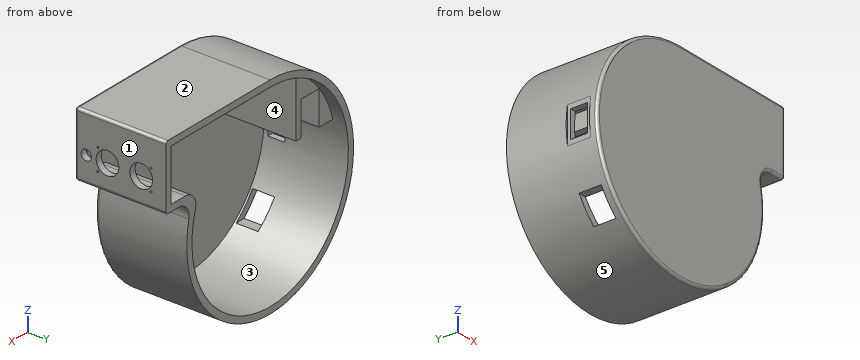
```python
from build123d import *

# Parameters (mm, degrees)
BOSS_EXTRUDE1_DEPTH     = 70
SHELL1_T                = -5
SKETCH3_R               = 8.75
SKETCH3_R_2             = 0.75
SKETCH3_R_3             = 4
CUT_EXTRUDE1_DEPTH      = 5
CUT_EXTRUDE2_REACH      = 147.945
CUT_EXTRUDE2_END_RADIUS = 80
SKETCH4_W               = 17
SKETCH4_H               = 17
SKETCH4_W_2             = 21
SKETCH4_H_2             = 13
CUT_EXTRUDE3_DEPTH      = 146.945195193
CUT_EXTRUDE3_DEPTH_BACK = 146.945195193
SKETCH5_W               = 2.5
SKETCH5_H               = 18
BOSS_EXTRUDE3_DEPTH     = 55
FILLET1_R               = 10
FILLET2_R               = 2


with BuildPart() as part:
    # Sketch1 → Boss-Extrude1 (new body)
    with BuildSketch(Plane(origin=(0, 0, 0), x_dir=(1, 0, 0), z_dir=(0, 1, 0))):
        with BuildLine():
            Line((0, -80), (100, -80))
            Line((100, -80), (100, -30))
            Line((100, -30), (74.161984871, -30))
            ThreePointArc((74.161984871, -30), (-44.72135955, 66.332495807), (0, -80))
        make_face()
    extrude(amount=BOSS_EXTRUDE1_DEPTH)

    # Shell1
    shell1_openings = [part.faces().sort_by_distance(p)[0] for p in [
        (7.618956149, 70, 6.200850369),
    ]]
    offset(amount=SHELL1_T, openings=shell1_openings, kind=Kind.INTERSECTION)

    # Sketch3 → Cut-Extrude1 (cut)
    with BuildSketch(Plane(origin=(100, 0, 0), x_dir=(0, 0, -1), z_dir=(1, 0, 0))):
        with Locations((-50, 25)):
            Circle(SKETCH3_R)
        with Locations((-50, 51)):
            Circle(SKETCH3_R)
        with Locations((-41.75, 58.5)):
            Circle(SKETCH3_R_2)
        with Locations((-41.75, 17.5)):
            Circle(SKETCH3_R_2)
        with Locations((-58.25, 17.5)):
            Circle(SKETCH3_R_2)
        with Locations((-58.25, 58.5)):
            Circle(SKETCH3_R_2)
        with Locations((-50, 8.65)):
            Circle(SKETCH3_R_3)
    extrude(amount=-CUT_EXTRUDE1_DEPTH, mode=Mode.SUBTRACT)

    # Cut-Extrude2: up to this cylinder (the profile starts inside it)
    cut_extrude2_end = Plane(origin=(0, 15, 0), z_dir=(0, -1, 0)) * Cylinder(CUT_EXTRUDE2_END_RADIUS, 456.89, mode=Mode.PRIVATE)
    # Sketch4 → Cut-Extrude2 (cut, up to the surface)
    with BuildSketch(Plane(origin=(0, 0, 0), x_dir=(0, 0, -1), z_dir=(1, 0, 0)), mode=Mode.PRIVATE) as cut_extrude2_sk1:
        with Locations((50.5, 15)):
            Rectangle(SKETCH4_W, SKETCH4_H)
    cut_extrude2_tool1 = extrude(cut_extrude2_sk1.sketch, amount=-CUT_EXTRUDE2_REACH, mode=Mode.PRIVATE) & cut_extrude2_end
    add(cut_extrude2_tool1.solids().sort_by_distance((0, 15, -50.5))[0], mode=Mode.SUBTRACT)
    # Sketch4 → Cut-Extrude2 (cut, up to the surface)
    with BuildSketch(Plane(origin=(0, 0, 0), x_dir=(0, 0, -1), z_dir=(1, 0, 0)), mode=Mode.PRIVATE) as cut_extrude2_sk2:
        with Locations((0, 15)):
            Rectangle(SKETCH4_W_2, SKETCH4_H_2)
    cut_extrude2_tool2 = extrude(cut_extrude2_sk2.sketch, amount=-CUT_EXTRUDE2_REACH, mode=Mode.PRIVATE) & cut_extrude2_end
    add(cut_extrude2_tool2.solids().sort_by_distance((0, 15, 0))[0], mode=Mode.SUBTRACT)

    # Sketch5 → Cut-Extrude3 (cut, two sides: drawn at the far end of the back side and taken through both)
    with BuildSketch(Plane.XY.offset(-CUT_EXTRUDE3_DEPTH_BACK)):
        with Locations((-79.998342826, 15)):
            Rectangle(SKETCH5_W, SKETCH5_H)
    extrude(amount=CUT_EXTRUDE3_DEPTH + CUT_EXTRUDE3_DEPTH_BACK, mode=Mode.SUBTRACT)

    # Sketch6 → Boss-Extrude3 (add)
    with BuildSketch(Plane(origin=(0, 5, 0), x_dir=(1, 0, 0), z_dir=(0, 1, 0))):
        with BuildLine():
            Line((-72.5176701, -19.136026841), (-59.5176701, -19.136026841))
            Line((-59.5176701, -19.136026841), (-59.5176701, -45.636026841))
            Line((-59.5176701, -45.636026841), (-42.0176701, -45.636026841))
            Line((-42.0176701, -45.636026841), (-42.0176701, -19.136026841))
            Line((-42.0176701, -19.136026841), (-37.0176701, -19.136026841))
            Line((-37.0176701, -19.136026841), (-37.0176701, -65.228000892))
            Line((-37.0176701, -65.228000892), (-37.0176701, -67.228000892))
            ThreePointArc((-37.0176701, -67.228000892), (-61.280154536, -47.480406071), (-74.5176701, -19.136026841))
            Line((-74.5176701, -19.136026841), (-72.5176701, -19.136026841))
        make_face()
    extrude(amount=BOSS_EXTRUDE3_DEPTH)

    # Fillet1
    fillet1_edges = [part.edges().sort_by_distance(p)[0] for p in [
        (66.332495807, 37.5, 35),
        (74.161984871, 35, 30),
    ]]
    fillet(fillet1_edges, radius=FILLET1_R)

    # Fillet2
    fillet2_edges = [part.edges().sort_by_distance(p)[0] for p in [
        (-49.888765157, 0, -62.538876798),
        (79.932284274, 0, 26.236095645),
        (93.874821937, 0, 30),
        (100, 0, 55),
        (50, 0, 80),
        (100, 35, 30),
        (100, 35, 80),
    ]]
    fillet(fillet2_edges, radius=FILLET2_R)


solid = part.part
```
Part model, mm, in its own coordinate system. Face numbers are marked on the shaded views. A direction names the side the tool comes from. Round coordinates to 2 decimals unless told otherwise and drop trailing zeros. Loops run counter-clockwise (first coordinate to the right, second up) from the corner with the lowest first, then second, coordinate; pieces in that order, holes last.
Item 1: 3-axis set-ups, long thin cutter, end or side, ignore diameter. For the marked faces 4 and 5: which of +Z, -Z, +X, -X, +Y, -Y reach the whole face in a straight line?
Item 2: Cut at B-B, the plane y = 48.5. Give the cut face in (x, z).
Item 3: Drop flat-ended pins along their axis: P1, Ø9, axis at x = -50, y = 26.5, coming from the -Z side; P2, Ø5, axis at x = 32.5, z = 1, coming from the +Y side; P3, Ø7, axis at y = 8.65, z = 50, coming from the -X side. Give the stop position or say it passes through.
Item 4: Cut at A-A, the plane y = 36.5. Give the cut face in (x, z).
Item 5: Cut at C-C, the plane y = 62.5. Give the cut face in (x, z), then the cut area to 3 significant figures.
Item 6: Mould opens along Z. For the marked faces 1, 2 and 3 say: +Z half, -Z half, draft (parallel to the pull), parting line (faces both ways), or undercut.
Item 7: Drill centre lines: line 1 (Y direction, x = 98, z = 50); line 2 (Z direction, x = 97, y = 58); line 3 (Z direction, x = 96.75, y = 8.65). Where is each one in solid material? Low to high.
A:
1. face 4: +Y
1. face 5: +Y, -Y
2. outline: (-72.52, 19.14) - (-59.52, 19.14) - (-59.52, 45.64) - (-42.02, 45.64) - (-42.02, 19.14) - (-37.02, 19.14) - (-37.02, 65.23) arc R75 cw to (0, 75) - (95, 75) - (95, 58.39) - (100, 58.39) - (100, 78) arc R2 ccw to (98, 80) - (0, 80) arc R80 ccw (long way) to (78, 17.78) arc R10 cw to (87.75, 30) - (98, 30) arc R2 ccw to (100, 32) - (100, 41.61) - (95, 41.61) - (95, 35) - (81.24, 35) arc R10 ccw to (71.68, 22.06) arc R75 cw (long way) to start
3. P1: stops at z = -65.8
3. P2: stops at y = 5
3. P3: stops at x = -65.1
4. outline: (0, 80) arc R80 ccw (long way) to (78, 17.78) arc R10 cw to (87.75, 30) - (98, 30) arc R2 ccw to (100, 32) - (100, 78) arc R2 ccw to (98, 80) - close; hole (-72.52, 19.14) arc R75 ccw (long way) to (71.68, 22.06) arc R10 cw to (81.24, 35) - (95, 35) - (95, 75) - (0, 75) arc R75 ccw to (-37.02, 65.23) - (-37.02, 19.14) - (-42.02, 19.14) - (-42.02, 45.64) - (-59.52, 45.64) - (-59.52, 19.14) - close
5. outline: (0, 80) arc R80 ccw (long way) to (78, 17.78) arc R10 cw to (87.75, 30) - (98, 30) arc R2 ccw to (100, 32) - (100, 78) arc R2 ccw to (98, 80) - close; hole (0, 75) arc R75 ccw (long way) to (71.68, 22.06) arc R10 cw to (81.24, 35) - (95, 35) - (95, 75) - close
5. area: 2,830 mm2
6. face 1: draft
6. face 2: +Z half
6. face 3: undercut
7. line 1: y = 0 to 4.65, 12.65 to 16.25, 33.75 to 42.25, 59.75 to 70
7. line 2: z = 30 to 41.19, 42.31 to 44.75, 55.25 to 57.69, 58.81 to 80
7. line 3: z = 30 to 46, 54 to 80
